```python
from build123d import *

# Parameters (mm, degrees)
SKETCH9_R           = 5
BOSS_EXTRUDE5_DEPTH = 5
SKETCH10_R          = 2.5
CUT_EXTRUDE5_DEPTH  = 46.760244755
SKETCH11_R          = 6
CUT_EXTRUDE6_DEPTH  = 8
SKETCH12_R          = 1.5
CUT_EXTRUDE7_DEPTH  = 36.411862419


with BuildPart() as part:
    # Sketch9 → Boss-Extrude5 (new, symmetric)
    with BuildSketch(Plane(origin=(0, 0, 0), x_dir=(1, 0, 0), z_dir=(0, 1, 0))):
        Polygon((12, 7.5), (12, -7.5), (25, -7.5), (25, -15), (15, -15), (15, -23), (-15, -23), (-15, -15), (-25, -15), (-25, -7.5), (-12, -7.5), (-12, 7.5), (-25, 7.5), (-25, 15), (-15, 15), (-15, 23), (15, 23), (15, 15), (25, 15), (25, 7.5), align=None)
        with Locations(Location((0, 0, 0), (0, 0, 270))):
            Circle(SKETCH9_R, mode=Mode.SUBTRACT)
    extrude(amount=BOSS_EXTRUDE5_DEPTH, both=True)

    # Sketch10 → Cut-Extrude5 (cut, through all)
    with BuildSketch(Plane(origin=(0, 0, -15), x_dir=(-1, 0, 0), z_dir=(0, 0, -1))):
        with Locations((20, 0)):
            Circle(SKETCH10_R)
        with Locations((-20, 0)):
            Circle(SKETCH10_R)
    extrude(amount=-CUT_EXTRUDE5_DEPTH, mode=Mode.SUBTRACT)

    # Sketch11 → Cut-Extrude6 (cut)
    with BuildSketch(Plane.XZ.offset(5)):
        with Locations(Location((0, 0, 0), (0, 0, 270))):
            Circle(SKETCH11_R)
    extrude(amount=-CUT_EXTRUDE6_DEPTH, mode=Mode.SUBTRACT)

    # Sketch12 → Cut-Extrude7 (cut, through all)
    with BuildSketch(Plane(origin=(0, 5, 0), x_dir=(1, 0, 0), z_dir=(0, 1, 0))):
        with Locations(Location((10, 19, 0), (0, 0, 270))):
            Circle(SKETCH12_R)
        with Locations(Location((-10, 19, 0), (0, 0, 90))):
            Circle(SKETCH12_R)
        with Locations(Location((10, -19, 0), (0, 0, 90))):
            Circle(SKETCH12_R)
        with Locations(Location((-10, -19, 0), (0, 0, 270))):
            Circle(SKETCH12_R)
    extrude(amount=-CUT_EXTRUDE7_DEPTH, mode=Mode.SUBTRACT)


solid = part.part
```
Input: part model. Units: mm. Frame: model coordinates. A direction names the side the tool comes from. Round coordinates to 2 decimals unless told otherwise and drop trailing zeros. Loops run counter-clockwise (first coordinate to the right, second up) from the corner with the lowest first, then second, coordinate; pieces in that order, holes last. Notation, with made-up numbers: (59, -3) -> (67, -3) arc R27 cw to (67, 15) -> close; hole circle Ø1 at (84, 41.25). An arc over 180 degrees is marked (long way). One line per item, written item: value.
(1) Section B-B (z = 0). Return the cut outline in (x, y), plus the area to 3 significant figures.
Geometry check:
outline: (-12, -5) -> (-6, -5) -> (-6, 3) -> (-5, 3) -> (-5, 5) -> (-12, 5) -> close; (5, 3) -> (6, 3) -> (6, -5) -> (12, -5) -> (12, 5) -> (5, 5) -> close
area: 124 mm2
(2) Set-up query: faces 5 (the face through (17, 0, -7.5)), 6 (the face through (15, 0, 19)), 7 (the face through (4, 3, 4)), 8 (the face through (-15, 0, -19)). Return all of +Z, -Z, +X, -X, +Y, -Y with unobstructed straight access to the full face (end or side cutting, diameter ignored); none if empty.
Geometry check:
face 5: +X, +Y, -Y
face 6: +Z, +X, +Y, -Y
face 7: -Y
face 8: -Z, -X, +Y, -Y
(3) Section A-A (x = -13). Return the cut outline in (y, z), plus the area to 3 significant figures.
Geometry check:
outline: (-5, -23) -> (5, -23) -> (5, -7.5) -> (-5, -7.5) -> close; (-5, 7.5) -> (5, 7.5) -> (5, 23) -> (-5, 23) -> close
area: 310 mm2
(4) Pin query (flat end, axial travel): pin 1 (2.5 mm diameter, centred on y = 1, z = -18.5, fed in from -X); pin 2 (3 mm diameter, centred on x = 19, y = -2.5, fed in from -Z); pin 3 (4 mm diameter, centred on y = 0, z = -18, fed in from +X). Return the tip coordinate at first contact, or that it passes through.
Geometry check:
pin 1: x = -15
pin 2: z = -15
pin 3: x = 15
(5) Section D-D (x = 10). Return the cut outline in (y, z).
Geometry check:
outline: (-5, -23) -> (5, -23) -> (5, -20.5) -> (-5, -20.5) -> close; (-5, -17.5) -> (5, -17.5) -> (5, 17.5) -> (-5, 17.5) -> close; (-5, 20.5) -> (5, 20.5) -> (5, 23) -> (-5, 23) -> close
(6) Section C-C (y = -3.75). Return the cut outline in (x, z), plus the area to 3 significant figures.
Geometry check:
outline: (-25, -15) -> (-15, -15) -> (-15, -23) -> (15, -23) -> (15, -15) -> (25, -15) -> (25, -7.5) -> (12, -7.5) -> (12, 7.5) -> (25, 7.5) -> (25, 15) -> (15, 15) -> (15, 23) -> (-15, 23) -> (-15, 15) -> (-25, 15) -> (-25, 7.5) -> (-12, 7.5) -> (-12, -7.5) -> (-25, -7.5) -> close; hole circle Ø3 at (-10, -19); hole circle Ø3 at (-10, 19); hole circle Ø12 at (0, 0); hole circle Ø3 at (10, -19); hole circle Ø3 at (10, 19)
area: 1,450 mm2
(7) Mould query, pull axis X, two halves, no side actions, for faces 1 (the face through (0, 0, 23)), 2 (the face through (12, 0, 0)), 3 (the face through (10.07, 0.07, -20.5)), 4 (the face through (-12, 0, 0)). Classes: pulls with the +X half, pulls with the -X half, needs draft (parallel to the pull), parting line crosses it, or undercut.
Geometry check:
face 1: needs draft
face 2: pulls with the +X half
face 3: undercut
face 4: pulls with the -X half
(8) Material intervals for line 1 (X direction, y = -0.25, z = -19); line 2 (X direction, y = 0.25, z = -9.5); line 3 (X direction, y = 4.1, z = 0), sorted ascending. Write a range as [from, to].
Geometry check:
line 1: [-15, -11.5], [-8.5, 8.5], [11.5, 15]
line 2: [-25, -22.49], [-17.51, 17.51], [22.49, 25]
line 3: [-12, -5], [5, 12]
